Geometry check sheet. Reference: drawing and pictorial views, mm from the part's lowest x, y, z. A direction names the side the tool comes from. Coordinates: 2 decimals unless noted, no trailing zeros. Write each loop counter-clockwise with the first axis right and the second up, starting at its lowest first coordinate (ties: lowest second). Pieces come first, ordered by that corner, then holes. Notation, with made-up numbers: (54.25, 13) -> (71.25, 13) arc R24 cw to (71.25, 46) -> close; hole circle Ø3 at (-11, 33). An arc over 180 degrees is marked (long way). Answer in a Markdown table with one row per item.
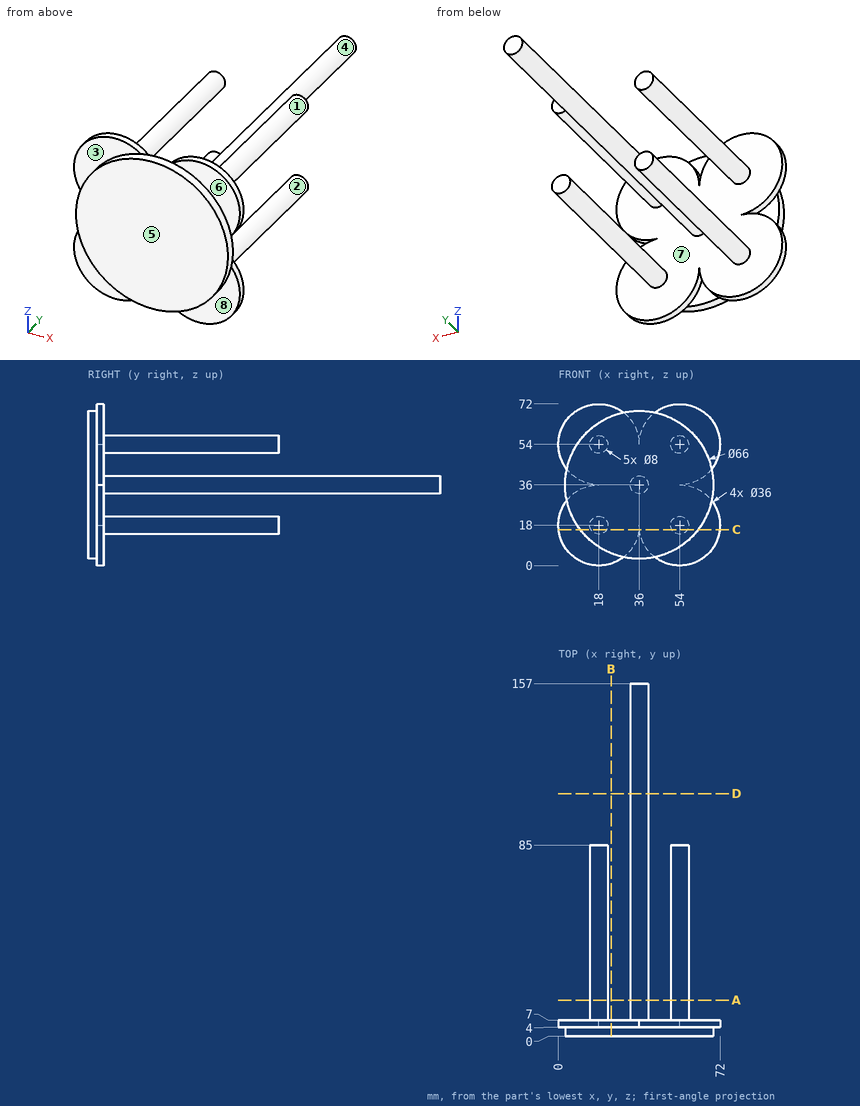
1. Section check A-A, the plane y = 16. Record the boundary of the cut face in (x, z).
Geometry says:
| item | result |
|---|---|
| outline | circle Ø8 at (18, 18); circle Ø8 at (18, 54); circle Ø8 at (36, 36); circle Ø8 at (54, 18); circle Ø8 at (54, 54) |
2. Tool access check on the marked faces 5, 6, 7 and 8. Record the directions out of +Z, -Z, +X, -X, +Y, -Y that give a thin tool (end or side, any length) a straight path to the whole face; none if there is none.
Geometry says:
| item | result |
|---|---|
| face 5 | +Z, -Z, +X, -X, -Y |
| face 6 | +Z, +X, -Y |
| face 7 | +Y |
| face 8 | -Z, +X, -Y |
3. Section check B-B, the plane x = 23.5. Record the boundary of the cut face in (y, z).
Geometry says:
| item | result |
|---|---|
| outline | (0, 5.46) -> (4, 5.46) -> (4, 0.86) -> (7, 0.86) -> (7, 71.14) -> (4, 71.14) -> (4, 66.54) -> (0, 66.54) -> close |
4. Depth check by flat-ended pin: P1, Ø2, axis at x = 37, y = 46, coming from the +Z side; P2, Ø2.5, axis at x = 55, z = 55.5, coming from the +Y side; P3, Ø7, axis at x = 37, z = 63.5, coming from the +Y side; P4, Ø8.5, axis at x = 63, z = 54.5, coming from the -Y side. Enter the tip coordinate at first touch or a pass-through.
Geometry says:
| item | result |
|---|---|
| P1 | z = 40 |
| P2 | y = 85 |
| P3 | y = 7 |
| P4 | y = 0 |
5. Section check C-C, the plane z = 16. Record the boundary of the cut face in (x, y).
Geometry says:
| item | result |
|---|---|
| outline | (0.11, 4) -> (9.75, 4) -> (9.75, 0) -> (62.25, 0) -> (62.25, 4) -> (71.89, 4) -> (71.89, 7) -> (57.46, 7) -> (57.46, 85) -> (50.54, 85) -> (50.54, 7) -> (36.11, 7) -> (36.11, 4) -> (35.89, 4) -> (35.89, 7) -> (21.46, 7) -> (21.46, 85) -> (14.54, 85) -> (14.54, 7) -> (0.11, 7) -> close |
6. Section check D-D, the plane y = 108. Record the boundary of the cut face in (x, z), plus the area to 3 significant figures.
Geometry says:
| item | result |
|---|---|
| outline | circle Ø8 at (36, 36) |
| area | 50.3 mm^2 |
7. Mould release check, pull along X, two halves, no side actions. Record for the marked faces 1, 2, 3 and 4: released by +X, released by -X, zero draft, split by the parting line, or undercut.
Geometry says:
| item | result |
|---|---|
| face 1 | undercut |
| face 2 | undercut |
| face 3 | zero draft |
| face 4 | split by the parting line |
8. Thickness scan on line 1 (Z direction, x = 17.5, y = 32.5); line 2 (X direction, y = 32.5, z = 54); line 3 (Y direction, x = 13, z = 10). Record the ranges inside material, lowest first. Write a range as from..to.
Geometry says:
| item | result |
|---|---|
| line 1 | 14.03..21.97, 50.03..57.97 |
| line 2 | 14..22, 50..58 |
| line 3 | 4..7 |
